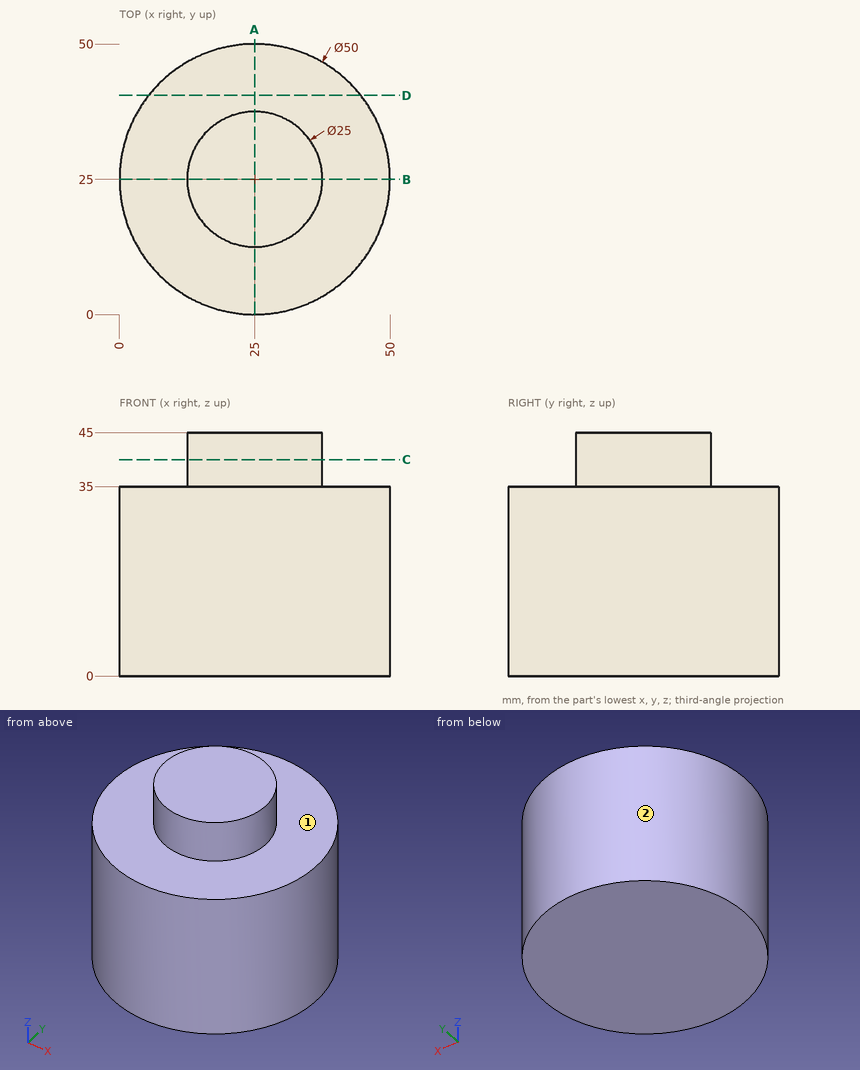
Can you work these out from the drawing? Everything is in mm from the part's minimum corner. A direction names the side the tool comes from. Round coordinates to 2 decimals unless told otherwise and drop trailing zeros. Order: outer loops, then holes, each group sorted by start corner. A loop starts at its lowest first (then second) coordinate and runs counter-clockwise, first axis right, second up. Notation, with made-up numbers: (-18.5, 43.25) - (39.5, 43.25) arc R31 cw to (39.5, 77.25) - close; hole circle Ø7 at (24.5, 31). An arc over 180 degrees is marked (long way). Answer in a Markdown table with one row per item.
(1) Suppose I cut it at D-D, the plane y = 40.5. Please give me the cut outline in (x, z).
From the geometry:
| item | result |
|---|---|
| outline | (5.38, 0) - (44.62, 0) - (44.62, 35) - (5.38, 35) - close |
(2) Suppose I cut it at A-A, the plane x = 25. Please give me the cut outline in (y, z).
From the geometry:
| item | result |
|---|---|
| outline | (0, 0) - (50, 0) - (50, 35) - (37.5, 35) - (37.5, 45) - (12.5, 45) - (12.5, 35) - (0, 35) - close |
(3) Suppose I cut it at C-C, the plane z = 40. Please give me the cut outline in (x, y).
From the geometry:
| item | result |
|---|---|
| outline | circle Ø25 at (25, 25) |
(4) For P1, Ø10, axis at x = 35.5, z = 33.5, coming from the -Y side; P2, Ø3, axis at x = 12, z = 23.5, coming from the -Y side; P3, Ø4, axis at x = 35.5, z = 24, coming from the -Y side, each with a flat end and sliding along its axis, tell me the tip position at first contact or that it passes through.
From the geometry:
| item | result |
|---|---|
| P1 | stops at y = 0.61 |
| P2 | stops at y = 2.8 |
| P3 | stops at y = 1.49 |
(5) Which directions (+Z, -Z, +X, -X, +Y, -Y) give clear straight access to the entire face, cutting with the end or side of a thin tool? Please do the marked faces 1 and 2.
From the geometry:
| item | result |
|---|---|
| face 1 | +Z |
| face 2 | +Z, -Z |
(6) Please list where these lines run through material, in increasing order: L1, parallel to Z at x = 12.5, y = 24; L2, parallel to X at y = 16.5, z = 21; L3, parallel to Y at x = 25, z = 11. Write a range as from..to.
From the geometry:
| item | result |
|---|---|
| L1 | z = 0..35 |
| L2 | x = 1.49..48.51 |
| L3 | y = 0..50 |
